Verification items for the finished model (mm, model axes). A direction names the side the tool comes from. Coordinates: 2 decimals unless noted, no trailing zeros. Write each loop counter-clockwise with the first axis right and the second up, starting at its lowest first coordinate (ties: lowest second). Pieces come first, ordered by that corner, then holes. Notation, with made-up numbers: (63, 37.25) - (98, 37.25) arc R27 cw to (98, 75.25) - close; hole circle Ø8 at (-14, 3.5). An arc over 180 degrees is marked (long way). Answer as CSV lines item,"result". Start each with the question number.
```python
from build123d import *

# Parameters (mm, degrees)
SKETCH1_W           = 9
SKETCH1_H           = 40
BOSS_EXTRUDE1_DEPTH = 2.5
BOSS_EXTRUDE2_START = -5.25
SKETCH2_R           = 2.5
BOSS_EXTRUDE2_DEPTH = 9.5
SKETCH3_R           = 1.5
CUT_EXTRUDE1_DEPTH  = 42.919565837
SKETCH4_R           = 2.875
CUT_EXTRUDE2_DEPTH  = 5.25
CUT_EXTRUDE3_START  = -14.75
SKETCH4_2_R         = 2.875
CUT_EXTRUDE3_DEPTH  = 5.25
SKETCH5_R           = 1
CUT_EXTRUDE4_DEPTH  = 42.695323479
CHAMFER1_SIZE       = 1.5
CHAMFER2_SIZE       = 1.5
SKETCH7_W           = 6.5
SKETCH7_H           = 0.2
CUT_EXTRUDE5_DEPTH  = 42.919565837


with BuildPart() as part:
    # Sketch1 → Boss-Extrude1 (new body)
    with BuildSketch(Plane(origin=(0, 0, 0), x_dir=(1, 0, 0), z_dir=(0, 1, 0))):
        with Locations((-4.5, 20)):
            Rectangle(SKETCH1_W, SKETCH1_H)
    extrude(amount=BOSS_EXTRUDE1_DEPTH)

    # Sketch2 → Boss-Extrude2 (add)
    with BuildSketch(Plane.XY.offset(BOSS_EXTRUDE2_START)):
        with Locations((-9, 2.5)):
            Circle(SKETCH2_R)
    boss_extrude2 = extrude(amount=-BOSS_EXTRUDE2_DEPTH)

    # Sketch3 → Cut-Extrude1 (cut, through all)
    with BuildSketch(Plane.XY):
        with Locations((-9, 2.5)):
            Circle(SKETCH3_R)
    cut_extrude1 = extrude(amount=-CUT_EXTRUDE1_DEPTH, mode=Mode.SUBTRACT)

    # Sketch4 → Cut-Extrude2 (cut)
    with BuildSketch(Plane.XY):
        with Locations((-9, 2.5)):
            Circle(SKETCH4_R)
    cut_extrude2 = extrude(amount=-CUT_EXTRUDE2_DEPTH, mode=Mode.SUBTRACT)

    # Sketch4<2> → Cut-Extrude3 (cut)
    with BuildSketch(Plane.XY.offset(CUT_EXTRUDE3_START)):
        with Locations((-9, 2.5)):
            Circle(SKETCH4_2_R)
    cut_extrude3 = extrude(amount=-CUT_EXTRUDE3_DEPTH, mode=Mode.SUBTRACT)

    # Mirror2: Boss-Extrude2, Cut-Extrude1, Cut-Extrude2, Cut-Extrude3 across plane
    add(boss_extrude2.mirror(Plane.XY.offset(-20)))
    add(cut_extrude1.mirror(Plane.XY.offset(-20)), mode=Mode.SUBTRACT)
    add(cut_extrude2.mirror(Plane.XY.offset(-20)), mode=Mode.SUBTRACT)
    add(cut_extrude3.mirror(Plane.XY.offset(-20)), mode=Mode.SUBTRACT)

    # Sketch5 → Cut-Extrude4 (cut, through all)
    with BuildSketch(Plane(origin=(0, 2.5, 0), x_dir=(1, 0, 0), z_dir=(0, 1, 0))):
        with Locations(Location((-3, 10, 0), (0, 0, 270))):
            Circle(SKETCH5_R)
    cut_extrude4 = extrude(amount=-CUT_EXTRUDE4_DEPTH, mode=Mode.SUBTRACT)

    # Mirror3: Cut-Extrude4 across plane
    add(cut_extrude4.mirror(Plane.XY.offset(-20)), mode=Mode.SUBTRACT)

    # Chamfer1
    chamfer1_edges = [part.edges().sort_by_distance(p)[0] for p in [
        (-3, 2.5, -29),
    ]]
    chamfer(chamfer1_edges, length=CHAMFER1_SIZE)

    # Chamfer2
    chamfer2_edges = [part.edges().sort_by_distance(p)[0] for p in [
        (-3, 2.5, -11),
    ]]
    chamfer(chamfer2_edges, length=CHAMFER2_SIZE)

    # Sketch7 → Cut-Extrude5 (cut, through all)
    with BuildSketch(Plane.XY):
        with Locations((-3.25, 2.4)):
            Rectangle(SKETCH7_W, SKETCH7_H)
    extrude(amount=-CUT_EXTRUDE5_DEPTH, mode=Mode.SUBTRACT)


solid = part.part
```
1. Depth check by flat-ended pin: P1, Ø5, axis at x = -4.5, z = -13, coming from the +Y side; P2, Ø3, axis at x = -3, z = -10, coming from the -Y side; P3, Ø6, axis at x = -2, z = -35.5, coming from the +Y side; P4, Ø2, axis at x = -7.5, z = -4, coming from the +Y side. Enter the tip coordinate at first touch or a pass-through.
2. Cross-section at C-C (y = 1.9). Record the cut outline in (x, z), and give its area (3 significant figures).
3. Access from +Z, -Z, +X, -X, +Y, -Y to the whole of each face (thin tool, end or side, straight path). Record for faces 4 (the face through (-6.58, 0.95, -37.41)), 5 (the face through (-10, 1, -14.75)), 6 (the face through (-3, 2.3, -20)), 7 (the face through (-10, 1, -5.25)).
4. Cross-section at A-A (z = -30). Record the cut outline in (x, y).
5. Cross-section at B-B (x = -3). Record the cut outline in (y, z), and give its area (3 significant figures).
6. Cross-section at D-D (x = -10). Record the cut outline in (y, z), and give its area (3 significant figures).
7. Scan lines: line 1 along X through (y, z) = (2.5, -32.25); line 2 along Y through (x, z) = (-9, -6.5); line 3 along Z through (x, y) = (-8.5, 4.6). Record each from-to range of solid material in increasing order. Write a range as from..to.
8. Draft check along X on faces 1 (the face through (-11, 4, -30)), 2 (the face through (-10, 1, -34.75)), 3 (the face through (-3, 0.5, -29)). Enter one of: pulls with the +X half, pulls with the -X half, needs draft (parallel to the pull), parting line crosses it, or undercut.
Completed:
1,P1,"stops at y = 4"
1,P2,"stops at y = 0"
1,P3,"stops at y = 2.3"
1,P4,"stops at y = 1.08"
2,outline,"(-11.43, -34.75) - (-10.37, -34.75) - (-10.37, -25.25) - (-11.43, -25.25) - close; (-11.43, -14.75) - (-10.37, -14.75) - (-10.37, -5.25) - (-11.43, -5.25) - close; (-7.63, -34.75) - (-6.19, -34.75) - (-6.19, -40) - (0, -40) - (0, 0) - (-6.19, 0) - (-6.19, -5.25) - (-7.63, -5.25) - (-7.63, -14.75) - (-6.19, -14.75) - (-6.19, -25.25) - (-7.63, -25.25) - close; hole circle Ø3.8 at (-3, -30); hole circle Ø3.8 at (-3, -10)"
2,area,"272 mm2"
3,face 4,"-Z, -X, +Y"
3,face 5,"-X, +Y"
3,face 6,"+Z, -Z, +X, +Y"
3,face 7,"+Z, -X, +Y"
4,outline,"(-9, 0) - (-4, 0) - (-4, 1) - (-5.3, 2.3) - (-6.5, 2.3) - (-6.5, 2.5) arc R2.5 ccw (long way) to start; (-2, 0) - (0, 0) - (0, 2.3) - (-0.7, 2.3) - (-2, 1) - close; hole circle Ø3 at (-9, 2.5)"
5,outline,"(0, -40) - (2.3, -40) - (2.3, -32.3) - (1, -31) - (0, -31) - close; (0, -29) - (1, -29) - (2.3, -27.7) - (2.3, -12.3) - (1, -11) - (0, -11) - close; (0, -9) - (1, -9) - (2.3, -7.7) - (2.3, 0) - (0, 0) - close"
5,area,"79.4 mm2"
6,outline,"(0.21, -34.75) - (1.38, -34.75) - (1.38, -25.25) - (0.21, -25.25) - close; (0.21, -14.75) - (1.38, -14.75) - (1.38, -5.25) - (0.21, -5.25) - close; (3.62, -34.75) - (4.79, -34.75) - (4.79, -25.25) - (3.62, -25.25) - close; (3.62, -14.75) - (4.79, -14.75) - (4.79, -5.25) - (3.62, -5.25) - close"
6,area,"44.6 mm2"
7,line 1,"x = -11.5..-10.5, -7.5..-6.5"
7,line 2,"y = 0..1, 4..5"
7,line 3,"z = -34.75..-25.25, -14.75..-5.25"
8,face 1,"parting line crosses it"
8,face 2,"needs draft"
8,face 3,"undercut"
